Can you work these out from the model? Positions are in its coordinate system, mm. A direction names the side the tool comes from. Give positions to 0.01 mm unless a question says otherwise; leave off trailing zeros. Loops run counter-clockwise (first coordinate to the right, second up) from the corner with the lowest first, then second, coordinate; pieces in that order, holes last. Notation, with made-up numbers: M -1.75,-35 L 46.25,-35 A14 cw 46.25,-28 Z; hole C 84,9 d6. An arc over 180 degrees is marked long. One line per item, written item: value. Start each with the question number.
Solid Edge part; units mm, degrees
sketch "Sketch1" plane through (0, 0, 0) normal (0, 0, 1) x (1, 0, 0)
  line L0 (-118.5746, -18.7961) -> (131.4254, -18.7961)
  line L1 (131.4254, -18.7961) -> (131.4254, 231.2039)
  line L2 (131.4254, 231.2039) -> (-118.5746, 231.2039)
  line L3 (-118.5746, 231.2039) -> (-118.5746, -18.7961)
  dimension "D1" = 131.4254
  dimension "D2" = 118.5746
extrude "Protrusion1" add sketch "Sketch1" along normal blind 20
sketch "Sketch2" plane through (-18.5746, 131.2039, 20) normal (0, 0, 1) x (1, 0, 0)
  circle A0 centre (25, 55) radius 20
extrude "Cutout1" cut sketch "Sketch2" against normal through all
sketch "Sketch3" plane through (31.4254, 131.2039, 0) normal (0, 0, -1) x (1, 0, 0)
  line L0 (100, 150) -> (70, 150)
  line L1 (70, 150) -> (70, 100)
  line L2 (70, 100) -> (100, 100)
  line L3 (100, 100) -> (100, 150)
  line L4 (-60, 150) -> (-60, 100)
  line L5 (-60, 100) -> (-30, 100)
  line L6 (-30, 100) -> (-30, 150)
  line L7 (-30, 150) -> (-60, 150)
  dimension "D1" = 60
  dimension "D2" = 100
  dimension "D3" = 100
  dimension "D4" = 30
extrude "ExtrudedProtrusion_2" add sketch "Sketch3" along normal blind 120
sketch "Sketch4" plane through (31.4254, 131.2039, 20) normal (0, 0, 1) x (-1, 0, 0)
  line L0 (30, 100) -> (60, 100)
  line L1 (60, 100) -> (60, 150)
  line L2 (60, 150) -> (30, 150)
  line L3 (30, 150) -> (30, 100)
  line L4 (-100, 150) -> (-100, 100)
  line L5 (-100, 100) -> (-70, 100)
  line L6 (-70, 100) -> (-70, 150)
  line L7 (-70, 150) -> (-100, 150)
  dimension "D1" = 100
  dimension "D2" = 70
  dimension "D3" = 60
  dimension "D4" = 70
extrude "ExtrudedProtrusion_4" add sketch "Sketch4" along normal blind 80
sketch "Sketch5" plane through (131.4254, 86.2039, 10) normal (1, 0, 0) x (0, 0, -1)
  circle A0 centre (100, -80) radius 5
  circle A1 centre (-60, -80) radius 5
  dimension "D1" = 60
extrude "Cutout2" cut sketch "Sketch5" against normal through all
sketch "Sketch6" plane through (31.4253, 131.2038, 20) normal (0, 0, 1) x (-1, 0, 0)
  line L0 (-70, 150) -> (-70, 49)
  line L1 (-70, 49) -> (30, 49)
  line L2 (30, 49) -> (30, 150)
  line L3 (30, 150) -> (-70, 150)
  dimension "D1" = 30
extrude "Cutout3" cut sketch "Sketch6" against normal through all
sketch "Sketch7" plane through (6.4254, 106.2039, 0) normal (0, 0, -1) x (-1, 0, 0)
  line L0 (-97.9157, 32.4862) -> (-97.9157, 129.3887)
  line L1 (-97.9157, 129.3887) -> (-214.4606, 129.3887)
  line L2 (-214.4606, 129.3887) -> (-214.4606, 32.4862)
  line L3 (-214.4606, 32.4862) -> (-97.9157, 32.4862)
  line L4 (35, -125) -> (35, 35.407)
  line L5 (35, 35.407) -> (133.9057, 35.407)
  line L6 (133.9057, 35.407) -> (133.9057, -125)
  line L7 (133.9057, -125) -> (35, -125)
extrude "Cutout4" cut sketch "Sketch7" against normal through all
Q1. If we section it at B-B, the plane z = 70: Write out the boundary of the cut face in (x, y).
Q2. I need wall thicknesses on line 1 along Y through (x, z) = (114.5, 70); line 2 along X through (y, z) = (7, 18); line 3 along Y through (x, z) = (-10, -105). Which ranges of each line are inside material? Lowest first, please.
Q3. If we mould it in two halves opening along Z, with no side actions, what happens to faces 1 (the face through (116, -18.796, -12)), 2 (the face through (-13.36, 4.29, -94.62)), 3 (the face through (-13, 7, -120)), 4 (the face through (-14, 7, 100))? For each: released by +Z, released by -Z, zero draft, split by the parting line, or undercut.
Q4. For P1, Ø6, axis at y = 6.2, z = -90, coming from the -X side; P2, Ø22, axis at x = 75, z = 13.5, coming from the -Y side; P3, Ø6, axis at y = 188.5, z = 8, coming from the +X side; P4, Ø6, axis at x = -79.5, z = 9, coming from the -Y side, each with a flat end and sliding along its axis, tell me the tip position at first contact or that it passes through.
Q5. If we section it at D-D, the plane x = 115: Write out the boundary of the cut face in (y, z), plus the area to 3 significant figures.
Q6. If we section it at A-A, the plane z = -70.5: Write out the boundary of the cut face in (x, y), plus the area to 3 significant figures.
Q7. Which directions (+Z, -Z, +X, -X, +Y, -Y) give clear straight access to the entire face, cutting with the end or side of a thin tool? Please do faces 5 (the face through (52, 82.204, 10)), 6 (the face through (101.425, 6, -59)), 7 (the face through (116, 31.204, -59)), 8 (the face through (118, 138.69, 10)), 9 (the face through (-28.575, 25, -8)).
Response:
1. outline: M -28.57,-18.8 L 1.43,-18.8 L 1.43,1.2 L -28.57,1.2 Z; M -28.57,11.2 L 1.43,11.2 L 1.43,31.2 L -28.57,31.2 Z; M 101.43,-18.8 L 131.43,-18.8 L 131.43,1.2 L 101.43,1.2 Z; M 101.43,11.2 L 131.43,11.2 L 131.43,31.2 L 101.43,31.2 Z
2. line 1: -18.8 to 1.2, 11.2 to 31.2
2. line 2: -28.57 to 1.43, 101.43 to 131.43
2. line 3: -18.8 to 31.2
3. face 1: zero draft
3. face 2: undercut
3. face 3: released by -Z
3. face 4: released by +Z
4. P1: through
4. P2: y = 82.2
4. P3: x = 104.34
4. P4: y = 141.61
5. outline: M -18.8,-120 L 31.2,-120 L 31.2,0 L 138.69,0 L 138.69,20 L 31.2,20 L 31.2,100 L -18.8,100 Z; hole C 6.2,-90 d10; hole C 6.2,70 d10
5. area: 13,000 mm^2
6. outline: M -28.57,-18.8 L 1.43,-18.8 L 1.43,31.2 L -28.57,31.2 Z; M 101.43,-18.8 L 131.43,-18.8 L 131.43,31.2 L 101.43,31.2 Z
6. area: 3,000 mm^2
7. face 5: +Z, -Z, -Y
7. face 6: +Z, -Z, +Y, -Y
7. face 7: -Z, +X, -X, +Y
7. face 8: +Z, -Z, +X, +Y
7. face 9: +Z, -Z, -X, -Y
